```python
from build123d import *

# Parameters (mm, degrees)
ESQUISSE1_W             = 70
ESQUISSE1_H             = 70
BOSS_EXTRU_1_DEPTH      = 50
ESQUISSE2_W             = 123.137615707
ESQUISSE2_H             = 86.86411441
ENL_V_MAT_EXTRU_1_DEPTH = 217
D_GAGEMENT_M41_D        = 4.5
D_GAGEMENT_M121_D       = 13.5
D_GAGEMENT_M61_D        = 6.6


with BuildPart() as part:
    # Esquisse1 → Boss.-Extru.1 (new body)
    with BuildSketch(Plane.XY):
        Rectangle(ESQUISSE1_W, ESQUISSE1_H)
    extrude(amount=BOSS_EXTRU_1_DEPTH)

    # Esquisse2 → Enlèv. mat.-Extru.1 (cut)
    with BuildSketch(Plane(origin=(35, 0, 0), x_dir=(0, 0, -1), z_dir=(1, 0, 0))):
        with Locations((-66.568807854, 13.432057205)):
            Rectangle(ESQUISSE2_W, ESQUISSE2_H)
    extrude(amount=-ENL_V_MAT_EXTRU_1_DEPTH, mode=Mode.SUBTRACT)

    # Dégagement M41 (through all)
    with Locations(Plane(origin=(0, 0, 0), x_dir=(-1, 0, 0), z_dir=(0, 0, -1))):
        with Locations((-26.157577905, 0.946358973), (27.533117647, 0.946358973)):
            Hole(D_GAGEMENT_M41_D / 2)

    # Dégagement M121 (through all)
    with Locations(Plane(origin=(0, 0, 0), x_dir=(-1, 0, 0), z_dir=(0, 0, -1))):
        with Locations((0.875458958, -21.366395267)):
            Hole(D_GAGEMENT_M121_D / 2)

    # Dégagement M61 (through all)
    with Locations(Plane(origin=(0, -30, 0), x_dir=(1, 0, 0), z_dir=(0, 1, 0))):
        with Locations((-23.62027619, -19.231813592), (22.015174003, -19.231813592)):
            Hole(D_GAGEMENT_M61_D / 2)


solid = part.part
```
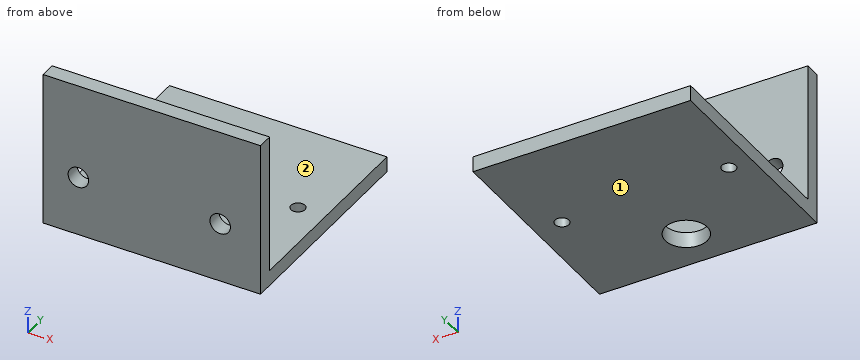
Model file for the job. Use its own axes, mm. Face numbers are marked on the shaded views. A direction names the side the tool comes from. Give positions to 0.01 mm unless a question says otherwise; leave off trailing zeros. Loops run counter-clockwise (first coordinate to the right, second up) from the corner with the lowest first, then second, coordinate; pieces in that order, holes last. Notation, with made-up numbers: (2, 22.25) -> (45, 22.25) arc R21 ccw to (45, 53.25) -> close; hole circle Ø10 at (57.25, 79.5). An arc over 180 degrees is marked (long way). Use CSV: the item, a comma, the result in double quotes. Start each with the question number.
1) Slice it at C-C on x = 12. Give the cut face in (y, z), plus the area to 3 significant figures.
2) Flat gauge pins, fed straight in: pin 1 Ø3 at (x, y) = (-6, 8.5) entering from +Z; pin 2 Ø10.5 at (x, z) = (22.02, 19.23) entering from +Y. Where does each tip first touch, or does it go through?
3) Slice it at A-A on x = 0. Give the cut face in (y, z).
4) Tool access for the marked faces 1 and 2: list every direction of +Z, -Z, +X, -X, +Y, -Y with a clear straight run to the whole face (end or side of a thin tool).
5) Slice it at D-D on z = 36. Give the cut face in (x, y), plus the area to 3 significant figures.
6) Wall check: line 1 (Y direction, x = 18.5, z = 30.5); line 2 (Z direction, x = -19, y = -11.5). Give the ranges that are in metal, low to high.
7) Slice it at B-B on y = -23.5. Give the cut face in (x, z).
Computed values:
1,outline,"(-35, 0) -> (35, 0) -> (35, 5) -> (-30, 5) -> (-30, 50) -> (-35, 50) -> close"
1,area,"575 mm^2"
2,pin 1,"stops at z = 5"
2,pin 2,"stops at y = -30"
3,outline,"(-35, 0) -> (-28.06, 0) -> (-28.06, 5) -> (-30, 5) -> (-30, 50) -> (-35, 50) -> close; (-14.67, 0) -> (35, 0) -> (35, 5) -> (-14.67, 5) -> close"
4,face 1,"-Z, +X, -X, +Y, -Y"
4,face 2,"+Z, +X, -X, +Y"
5,outline,"(-35, -35) -> (35, -35) -> (35, -30) -> (-35, -30) -> close"
5,area,"350 mm^2"
6,line 1,"y = -35 to -30"
6,line 2,"z = 0 to 5"
7,outline,"(-35, 0) -> (-7.28, 0) -> (-7.28, 5) -> (-35, 5) -> close; (5.53, 0) -> (35, 0) -> (35, 5) -> (5.53, 5) -> close"
